The drawing under review shows one solid part. Ordinate dimensions are in mm from its lowest x, y, z. A direction names the side the tool comes from. Give positions to 0.01 mm unless a question says otherwise; leave off trailing zeros. Write each loop counter-clockwise with the first axis right and the second up, starting at its lowest first coordinate (ties: lowest second). Pieces come first, ordered by that corner, then holes.
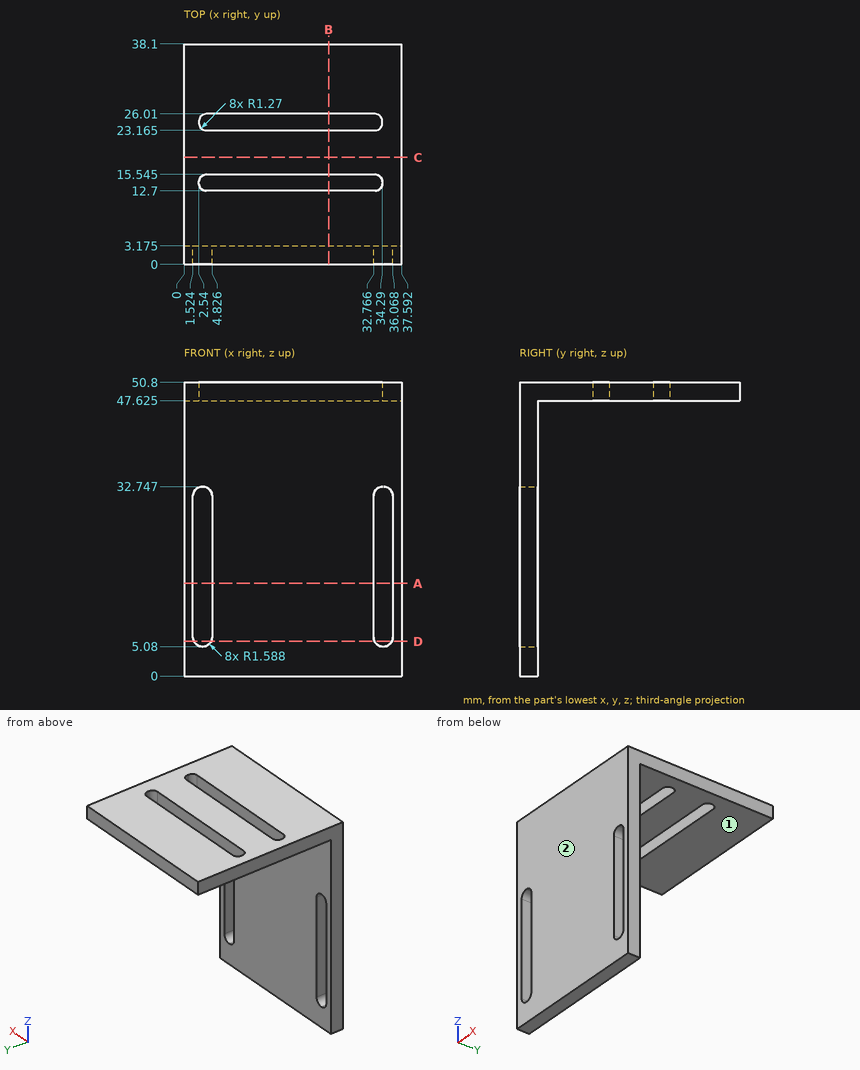
1) To check wall thickness, follow probe 1 along Z at (x, y) = (24, 8) (1 decimal); probe 2 along Y at (x, z) = (26, 30.5) (1 decimal). State the ranges of each line that lie inside material, in increasing order.
2) Consider section D-D, the plane z = 6. Give the boundary of the cut face in (x, y) (1 decimal).
3) Insertion check: pin 1 (4 mm diameter, centred on x = 27.5, z = 12.5, fed in from +Y) (1 decimal); pin 2 (10 mm diameter, centred on x = 31.5, y = 26.5, fed in from -Z) (1 decimal). Each pin has a flat end and moves straight along its axis. Give the tip position at first contact, or say it passes through.
4) Consider section C-C, the plane y = 18.5. Give the boundary of the cut face in (x, z) (1 decimal).
5) Consider section A-A, the plane z = 16. Give the boundary of the cut face in (x, y) (1 decimal).
6) Consider section B-B, the plane x = 25. Give the boundary of the cut face in (y, z) (1 decimal), then the cut area to 3 significant figures.
7) Tool access review of the marked faces 1 and 2: name each direction out of +Z, -Z, +X, -X, +Y, -Y from which nothing blocks a thin tool from reaching the whole face with its end or side.
Answer block:
1. probe 1: z = 47.6 to 50.8
1. probe 2: y = 0 to 3.2
2. outline: (0, 0) - (1.7, 0) - (1.7, 3.2) - (0, 3.2) - close; (4.7, 0) - (32.9, 0) - (32.9, 3.2) - (4.7, 3.2) - close; (35.9, 0) - (37.6, 0) - (37.6, 3.2) - (35.9, 3.2) - close
3. pin 1: stops at y = 3.2
3. pin 2: stops at z = 47.6
4. outline: (0, 47.6) - (37.6, 47.6) - (37.6, 50.8) - (0, 50.8) - close
5. outline: (0, 0) - (1.5, 0) - (1.5, 3.2) - (0, 3.2) - close; (4.8, 0) - (32.8, 0) - (32.8, 3.2) - (4.8, 3.2) - close; (36.1, 0) - (37.6, 0) - (37.6, 3.2) - (36.1, 3.2) - close
6. outline: (0, 0) - (3.2, 0) - (3.2, 47.6) - (12.7, 47.6) - (12.7, 50.8) - (0, 50.8) - close; (15.5, 47.6) - (23.2, 47.6) - (23.2, 50.8) - (15.5, 50.8) - close; (26, 47.6) - (38.1, 47.6) - (38.1, 50.8) - (26, 50.8) - close
6. area: 254 mm2
7. face 1: -Z, +X, -X, +Y
7. face 2: +Z, -Z, +X, -X, -Y
